Check sheet for the modelled part. Datum: model origin and axes. Units: mm. A direction names the side the tool comes from. Round coordinates to 2 decimals unless told otherwise and drop trailing zeros. Write each loop counter-clockwise with the first axis right and the second up, starting at its lowest first coordinate (ties: lowest second). Pieces come first, ordered by that corner, then holes. Notation, with made-up numbers: M 5,3 L 23,3 A26 ccw 23,29 Z; hole C -5.75,-9 d10. An arc over 180 degrees is marked long. Answer in a Markdown table with one row per item.
```python
from build123d import *

# Parameters (mm, degrees)
SKETCH_1_W          = 10
SKETCH_1_H          = 10
SKETCH_1_W_2        = 8
SKETCH_1_H_2        = 8
EXTRUDE_1_DEPTH     = 140
SKETCH_2_R          = 2.1
CUT_EXTRUDE_1_DEPTH = 141.445719052
SKETCH_3_R          = 2.1
CUT_EXTRUDE_2_DEPTH = 141.445719052


with BuildPart() as part:
    # ｽｹｯﾁ1 → 押し出し-薄板1 (new body)
    with BuildSketch(Plane(origin=(0, 0, 0), x_dir=(0, 0, -1), z_dir=(1, 0, 0))):
        Rectangle(SKETCH_1_W, SKETCH_1_H)
        Rectangle(SKETCH_1_W_2, SKETCH_1_H_2, mode=Mode.SUBTRACT)
    extrude(amount=EXTRUDE_1_DEPTH)

    # ｽｹｯﾁ2 → ｶｯﾄ - 押し出し1 (cut, through all)
    with BuildSketch(Plane(origin=(0, 5, 0), x_dir=(1, 0, 0), z_dir=(0, 1, 0))):
        with Locations(Location((5, 0, 0), (0, 0, 270))):
            Circle(SKETCH_2_R)
        with Locations(Location((135, 0, 0), (0, 0, 270))):
            Circle(SKETCH_2_R)
    extrude(amount=-CUT_EXTRUDE_1_DEPTH, mode=Mode.SUBTRACT)

    # ｽｹｯﾁ3 → ｶｯﾄ - 押し出し2 (cut, through all)
    with BuildSketch(Plane.XY.offset(5)):
        with Locations((40, 0)):
            Circle(SKETCH_3_R)
        with Locations((30, 0)):
            Circle(SKETCH_3_R)
        with Locations(Location((110, 0, 0), (0, 0, 90))):
            Circle(SKETCH_3_R)
        with Locations(Location((100, 0, 0), (0, 0, 90))):
            Circle(SKETCH_3_R)
    extrude(amount=-CUT_EXTRUDE_2_DEPTH, mode=Mode.SUBTRACT)


solid = part.part
```
1. Draft check along Y on faces 1 (the face through (69, -5, 0)), 2 (the face through (69, -4, 0)), 3 (the face through (101.863, 0.969, 4.507)), 4 (the face through (132.95, 4.51, -0.46)). Enter one of: +Y half, -Y half, draft (parallel to the pull), parting line (faces both ways), or undercut.
Found:
| item | result |
|---|---|
| face 1 | -Y half |
| face 2 | undercut |
| face 3 | undercut |
| face 4 | draft |
2. Section check A-A, the plane x = 110. Record the cut outline in (y, z), and give its area (3 significant figures).
Found:
| item | result |
|---|---|
| outline | M -5,-5 L -2.1,-5 L -2.1,-4 L -4,-4 L -4,4 L -2.1,4 L -2.1,5 L -5,5 Z; M 2.1,-5 L 5,-5 L 5,5 L 2.1,5 L 2.1,4 L 4,4 L 4,-4 L 2.1,-4 Z |
| area | 27.6 mm2 |
3. Section check B-B, the plane z = -0.5. Record the cut outline in (x, y), and give its area (3 significant figures).
Found:
| item | result |
|---|---|
| outline | M 0,-5 L 2.96,-5 L 2.96,-4 L 0,-4 Z; M 0,4 L 2.96,4 L 2.96,5 L 0,5 Z; M 7.04,-5 L 132.96,-5 L 132.96,-4 L 7.04,-4 Z; M 7.04,4 L 132.96,4 L 132.96,5 L 7.04,5 Z; M 137.04,-5 L 140,-5 L 140,-4 L 137.04,-4 Z; M 137.04,4 L 140,4 L 140,5 L 137.04,5 Z |
| area | 264 mm2 |
4. Section check C-C, the plane x = 71.5. Record the cut outline in (y, z), and give its area (3 significant figures).
Found:
| item | result |
|---|---|
| outline | M -5,-5 L 5,-5 L 5,5 L -5,5 Z; hole M -4,-4 L 4,-4 L 4,4 L -4,4 Z |
| area | 36.0 mm2 |
5. Scan lines: L1, parallel to X at y = -4.45, z = 0; L2, parallel to Y at x = 81, z = -3.75. Record each from-to range of solid material in increasing order.
Found:
| item | result |
|---|---|
| L1 | x = 0 to 2.9, 7.1 to 132.9, 137.1 to 140 |
| L2 | y = -5 to -4, 4 to 5 |
6. Access from +Z, -Z, +X, -X, +Y, -Y to the whole of each face (thin tool, end or side, straight path). Record for faces 5 (the face through (69, 0, 5)), 6 (the face through (69, 0, -4)).
Found:
| item | result |
|---|---|
| face 5 | +Z, +X, -X, +Y, -Y |
| face 6 | +X, -X |
7. Go/stop test with flat-tipped pins: pin 1 (4 mm diameter, centred on x = 110, y = 0, fed in from -Z); pin 2 (5 mm diameter, centred on y = -1, z = 3.5, fed in from +X). Record where each tip stops, or that it passes through.
Found:
| item | result |
|---|---|
| pin 1 | passes through |
| pin 2 | stops at x = 140 |
